Here's how the part is built. I have some questions about the finished solid (model axes, mm). A direction names the side the tool comes from. Round coordinates to 2 decimals unless told otherwise and drop trailing zeros. Order: outer loops, then holes, each group sorted by start corner. A loop starts at its lowest first (then second) coordinate and runs counter-clockwise, first axis right, second up.
```python
from build123d import *

# Parameters (mm, degrees)
SKETCH_1_W                       = 25
SKETCH_1_H                       = 35
SKETCH_1_R                       = 2.6
EXTRUDE_1_DEPTH                  = 4
EXTRUDE_2_DEPTH                  = 4
FILLET_1_R                       = 3.5
CUT_EXTRUDE_1_DEPTH              = 10
SKETCH_4_R                       = 2.1
CUT_EXTRUDE_2_DEPTH              = 10
PATTERN_CIRCULAR_1_COUNT         = 4
CUT_EXTRUDE_3_DEPTH              = 10
FILLET_2_R                       = 3
PATTERN_CIRCULAR_2_COUNT         = 4
FILLET_2_OF_PATTERN_CIRCULAR_2_R = 3
CUT_EXTRUDE_4_DEPTH              = 10
FILLET_3_R                       = 3


with BuildPart() as part:
    # 草图1 → 凸台-拉伸1 (new body)
    with BuildSketch(Plane(origin=(0, 0, 0), x_dir=(1, 0, 0), z_dir=(0, 1, 0))):
        Rectangle(SKETCH_1_W, SKETCH_1_H)
        with Locations(Location((7.5, 5, 0), (0, 0, 270))):
            Circle(SKETCH_1_R, mode=Mode.SUBTRACT)
        with Locations(Location((7.5, -5, 0), (0, 0, 270))):
            Circle(SKETCH_1_R, mode=Mode.SUBTRACT)
        with Locations(Location((-7.5, -10, 0), (0, 0, 270))):
            Circle(SKETCH_1_R, mode=Mode.SUBTRACT)
        with Locations(Location((-7.5, 10, 0), (0, 0, 270))):
            Circle(SKETCH_1_R, mode=Mode.SUBTRACT)
    extrude(amount=EXTRUDE_1_DEPTH)


with BuildPart() as body_2:
    # 草图2 → 凸台-拉伸2 (new body)
    with BuildSketch(Plane(origin=(0, 4, 0), x_dir=(1, 0, 0), z_dir=(0, 1, 0))):
        Polygon((-133.482, 27.5), (-78.482, 27.5), (-12.5, 17.5), (-12.5, -17.5), (-78.482, -27.5), (-133.482, -27.5), align=None)
    extrude(amount=-EXTRUDE_2_DEPTH)


with BuildPart() as part_1:
    add(part.part)

    # Combine 1: union body 2
    add(body_2.part)

    # 圆角1
    fillet_1_edges = [part_1.edges().sort_by_distance(p)[0] for p in [
        (-12.5, 2, -17.5),
        (-12.5, 2, 17.5),
        (-78.482, 2, 27.5),
        (-133.482, 2, 27.5),
        (-133.482, 2, -27.5),
        (-78.482, 2, -27.5),
    ]]
    fillet(fillet_1_edges, radius=FILLET_1_R)

    # 草图3 → 切除-拉伸1 (cut)
    with BuildSketch(Plane(origin=(0, 4, 0), x_dir=(1, 0, 0), z_dir=(0, 1, 0))):
        with BuildLine():
            ThreePointArc((-92.832, 0), (-100.949712864, 12.149015853), (-115.280454173, 9.298454173))
            Line((-115.280454173, 9.298454173), (-105.982, 0))
            Line((-105.982, 0), (-115.280454173, -9.298454173))
            ThreePointArc((-115.280454173, -9.298454173), (-100.949712864, -12.149015853), (-92.832, 0))
        make_face()
        with BuildLine():
            Line((-105.982, 0), (-115.280454173, 9.298454173))
            ThreePointArc((-115.280454173, 9.298454173), (-119.132, 0), (-115.280454173, -9.298454173))
            Line((-115.280454173, -9.298454173), (-105.982, 0))
        make_face()
        with BuildLine():
            ThreePointArc((-92.832, 0), (-100.949712864, 12.149015853), (-115.280454173, 9.298454173))
            Line((-115.280454173, 9.298454173), (-105.982, 0))
            Line((-105.982, 0), (-115.280454173, -9.298454173))
            ThreePointArc((-115.280454173, -9.298454173), (-100.949712864, -12.149015853), (-92.832, 0))
        make_face()
        with BuildLine():
            Line((-105.982, 0), (-115.280454173, 9.298454173))
            ThreePointArc((-115.280454173, 9.298454173), (-119.132, 0), (-115.280454173, -9.298454173))
            Line((-115.280454173, -9.298454173), (-105.982, 0))
        make_face()
    extrude(amount=-CUT_EXTRUDE_1_DEPTH, mode=Mode.SUBTRACT)

    # 草图4 → 切除-拉伸2 (cut)
    with BuildSketch(Plane(origin=(0, 4, 0), x_dir=(1, 0, 0), z_dir=(0, 1, 0))):
        with Locations(Location((-81.982, 24, 0), (0, 0, 270))):
            Circle(SKETCH_4_R)
    cut_extrude_2 = extrude(amount=-CUT_EXTRUDE_2_DEPTH, mode=Mode.SUBTRACT)

    # 阵列(圆周)1: 切除-拉伸2 ×4 about axis
    pattern_circular_1_axis = Axis((-105.982, 0, 0), (0, 1, 0))
    for i in range(1, PATTERN_CIRCULAR_1_COUNT):
        add(cut_extrude_2.rotate(pattern_circular_1_axis, i * 360 / PATTERN_CIRCULAR_1_COUNT), mode=Mode.SUBTRACT)

    # 草图5 → 切除-拉伸3 (cut)
    with BuildSketch(Plane(origin=(0, 4, 0), x_dir=(1, 0, 0), z_dir=(0, 1, 0))):
        with BuildLine():
            Line((-120.461424988, 10.943891082), (-128.482, 18.964466094))
            Line((-128.482, 18.964466094), (-128.482, -18.964466094))
            Line((-128.482, -18.964466094), (-120.461424988, -10.943891082))
            ThreePointArc((-120.461424988, -10.943891082), (-124.132, 0), (-120.461424988, 10.943891082))
        make_face()
    cut_extrude_3 = extrude(amount=-CUT_EXTRUDE_3_DEPTH, mode=Mode.SUBTRACT)

    # 圆角2
    fillet_2_edges = [part_1.edges().sort_by_distance(p)[0] for p in [
        (-120.461424988, 2, -10.943891082),
        (-120.461424988, 2, 10.943891082),
        (-128.482, 2, 18.964466094),
        (-128.482, 2, -18.964466094),
    ]]
    fillet(fillet_2_edges, radius=FILLET_2_R)

    # 阵列(圆周)2: 切除-拉伸3 ×4 about axis
    pattern_circular_2_axis = Axis((-105.982, 0, 0), (0, 1, 0))
    for i in range(1, PATTERN_CIRCULAR_2_COUNT):
        add(cut_extrude_3.rotate(pattern_circular_2_axis, i * 360 / PATTERN_CIRCULAR_2_COUNT), mode=Mode.SUBTRACT)

    # 圆角2 of 阵列(圆周)2
    fillet_2_of_pattern_circular_2_edges = [part_1.edges().sort_by_distance(p)[0] for p in [
        (-116.925891082, 2, 14.479424988),
        (-95.038108918, 2, 14.479424988),
        (-87.017533906, 2, 22.5),
        (-124.946466094, 2, 22.5),
        (-91.502575012, 2, 10.943891082),
        (-91.502575012, 2, -10.943891082),
        (-83.482, 2, -18.964466094),
        (-83.482, 2, 18.964466094),
        (-95.038108918, 2, -14.479424988),
        (-116.925891082, 2, -14.479424988),
        (-124.946466094, 2, -22.5),
        (-87.017533906, 2, -22.5),
    ]]
    fillet(fillet_2_of_pattern_circular_2_edges, radius=FILLET_2_OF_PATTERN_CIRCULAR_2_R)

    # 草图6 → 切除-拉伸4 (cut)
    with BuildSketch(Plane(origin=(0, 4, 0), x_dir=(1, 0, 0), z_dir=(0, 1, 0))):
        Polygon((-73.221259435, -18.460580976), (-49.753485721, 0.064081858), (-73.221259435, 18.634602448), align=None)
        Polygon((-45.719729218, 3.248192123), (-30.596936447, 15.18561067), (-67.961344653, 20.848429046), align=None)
        Polygon((-68.227570637, -20.88877732), (-30.500709207, -15.171026808), (-45.723561893, -3.124877792), align=None)
    extrude(amount=-CUT_EXTRUDE_4_DEPTH, mode=Mode.SUBTRACT)

    # 圆角3
    fillet_3_edges = [part_1.edges().sort_by_distance(p)[0] for p in [
        (-30.500709207, 2, 15.171026808),
        (-68.227570637, 2, 20.88877732),
        (-45.723561893, 2, 3.124877792),
        (-45.719729218, 2, -3.248192123),
        (-67.961344653, 2, -20.848429046),
        (-30.596936447, 2, -15.18561067),
        (-73.221259435, 2, 18.460580976),
        (-73.221259435, 2, -18.634602448),
        (-49.753485721, 2, -0.064081858),
    ]]
    fillet(fillet_3_edges, radius=FILLET_3_R)


solid = part_1.part
```
1. I'm going to push flat-ended pins straight in: P1, Ø2, axis at x = 2, y = 1.5, coming from the -Z side; P2, Ø2, axis at x = -2.5, y = 1, coming from the +Z side. Where does each tip first touch, or does it pass through?
Evaluation:
P1: stops at z = -17.5
P2: stops at z = 17.5
2. If we section it at C-C, the plane y = 2.7: State how many separate pieces and enclosed holes the cut face has, and give its area (3 significant figures).
Evaluation:
separate pieces: 1
enclosed holes: 16
area: 4,650 mm2
3. If we section it at A-A, the plane x = 7.5: Write out the boundary of the cut face in (y, z), and give its area (3 significant figures).
Evaluation:
outline: (0, -17.5) - (4, -17.5) - (4, -7.6) - (0, -7.6) - close; (0, -2.4) - (4, -2.4) - (4, 2.4) - (0, 2.4) - close; (0, 7.6) - (4, 7.6) - (4, 17.5) - (0, 17.5) - close
area: 98.4 mm2
4. On a 3-axis mill with a long thin cutter (end or side, diameter ignored), from which of +Z, -Z, +X, -X, +Y, -Y can I reach the whole of each face in a straight line? I mean faces 1 (the cylindrical face through (-51.59, 1.97, -0.1)), 2 (the flat face through (-59, 0, 12)). Say none if no direction works.
Evaluation:
face 1: +Y, -Y
face 2: +Z, -Z, +X, -X, -Y
5. If we section it at B-B, the plane x = -113: Write out the boundary of the cut face in (y, z).
Evaluation:
outline: (0, -27.5) - (4, -27.5) - (4, -22.5) - (0, -22.5) - close; (0, -16.74) - (4, -16.74) - (4, -11.12) - (0, -11.12) - close; (0, 11.12) - (4, 11.12) - (4, 16.74) - (0, 16.74) - close; (0, 22.5) - (4, 22.5) - (4, 27.5) - (0, 27.5) - close
6. If we mould it in two halves opening along X, with no side actions, what happens to faces 3 (the cylindrical face through (-45.747, 1.972, -4.072)), 4 (the flat face through (-45.03, 2.03, 22.43)), 5 (the flat face through (-105, 2, -27.5))? For each: released by +X, released by -X, zero draft, split by the parting line, or undercut.
Evaluation:
face 3: undercut
face 4: released by +X
face 5: zero draft
7. I need wall thicknesses on probe 1 along Z at (x, y) = (-106.5, 2.2); probe 2 along X at (y, z) = (0.35, -3.5); probe 3 along Z at (x, y) = (-104, 2.05). Which ranges of each line are inside material? Lowest first, please.
Evaluation:
probe 1: z = -27.5 to -22.5, -18.14 to -13.14, 13.14 to 18.14, 22.5 to 27.5
probe 2: x = -133.48 to -128.48, -123.79 to -118.66, -93.31 to -88.17, -83.48 to -73.22, -54.1 to 5.38, 9.62 to 12.5
probe 3: z = -27.5 to -22.5, -18.04 to -13, 13 to 18.04, 22.5 to 27.5
